from build123d import *

# Parameters (mm, degrees)
BOSS_EXTRUDE1_DEPTH = 4.4
SKETCH2_R           = 3.5
CUT_EXTRUDE1_DEPTH  = 1
SKETCH2_3_R         = 1.7
CUT_EXTRUDE2_DEPTH  = 35.625460286
BOSS_EXTRUDE2_DEPTH = 11.6
FILLET1_R           = 1
CUT_EXTRUDE3_DEPTH  = 5
SKETCH5_R           = 2.5
CUT_EXTRUDE4_DEPTH  = 11


with BuildPart() as part:
    # Sketch1 → Boss-Extrude1 (new body)
    with BuildSketch(Plane(origin=(0, 0, 0), x_dir=(1, 0, 0), z_dir=(0, 1, 0))):
        with BuildLine():
            Line((-11.25, 18), (11.25, 18))
            ThreePointArc((11.25, 18), (29.25, 0), (11.25, -18))
            Line((11.25, -18), (-11.25, -18))
            ThreePointArc((-11.25, -18), (-29.25, 0), (-11.25, 18))
        make_face()
    extrude(amount=BOSS_EXTRUDE1_DEPTH)

    # Sketch2 → Cut-Extrude1 (cut)
    with BuildSketch(Plane(origin=(0, 4.4, 0), x_dir=(1, 0, 0), z_dir=(0, 1, 0))):
        with Locations(Location((-24.25, 0, 0), (0, 0, 270))):
            Circle(SKETCH2_R)
        with Locations(Location((-11.25, 13, 0), (0, 0, 270))):
            Circle(SKETCH2_R)
        with Locations(Location((11.25, 13, 0), (0, 0, 270))):
            Circle(SKETCH2_R)
        with Locations(Location((24.25, 0, 0), (0, 0, 270))):
            Circle(SKETCH2_R)
        with Locations(Location((11.25, -13, 0), (0, 0, 270))):
            Circle(SKETCH2_R)
        with Locations(Location((-11.25, -13, 0), (0, 0, 270))):
            Circle(SKETCH2_R)
    extrude(amount=-CUT_EXTRUDE1_DEPTH, mode=Mode.SUBTRACT)

    # Sketch2<3> → Cut-Extrude2 (cut, through all)
    with BuildSketch(Plane(origin=(0, 4.4, 0), x_dir=(1, 0, 0), z_dir=(0, 1, 0))):
        with Locations(Location((-11.25, 13, 0), (0, 0, 270))):
            Circle(SKETCH2_3_R)
        with Locations(Location((-24.25, 0, 0), (0, 0, 270))):
            Circle(SKETCH2_3_R)
        with Locations(Location((-11.25, -13, 0), (0, 0, 270))):
            Circle(SKETCH2_3_R)
        with Locations(Location((11.25, -13, 0), (0, 0, 270))):
            Circle(SKETCH2_3_R)
        with Locations(Location((24.25, 0, 0), (0, 0, 270))):
            Circle(SKETCH2_3_R)
        with Locations(Location((11.25, 13, 0), (0, 0, 270))):
            Circle(SKETCH2_3_R)
    extrude(amount=-CUT_EXTRUDE2_DEPTH, mode=Mode.SUBTRACT)

    # Sketch3 → Boss-Extrude2 (add)
    with BuildSketch(Plane(origin=(0, 4.4, 0), x_dir=(1, 0, 0), z_dir=(0, 1, 0))):
        with BuildLine():
            Line((-11.25, 7.6), (11.25, 7.6))
            ThreePointArc((11.25, 7.6), (18.85, 0), (11.25, -7.6))
            Line((11.25, -7.6), (-11.25, -7.6))
            ThreePointArc((-11.25, -7.6), (-18.85, 0), (-11.25, 7.6))
        make_face()
    extrude(amount=BOSS_EXTRUDE2_DEPTH)

    # Fillet1
    fillet1_edges = [part.edges().sort_by_distance(p)[0] for p in [
        (29.25, 4.4, 0),
        (0, 4.4, -18),
        (-29.25, 4.4, 0),
        (-18.85, 4.4, 0),
        (0, 4.4, 7.6),
        (18.85, 4.4, 0),
        (0, 4.4, -7.6),
        (0, 4.4, 18),
    ]]
    fillet(fillet1_edges, radius=FILLET1_R)

    # Sketch4 → Cut-Extrude3 (cut)
    with BuildSketch(Plane(origin=(0, 16, 0), x_dir=(1, 0, 0), z_dir=(0, 1, 0))):
        with BuildLine():
            Line((-11.25, 5), (11.25, 5))
            ThreePointArc((11.25, 5), (16.25, 0), (11.25, -5))
            Line((11.25, -5), (-11.25, -5))
            ThreePointArc((-11.25, -5), (-16.25, 0), (-11.25, 5))
        make_face()
    extrude(amount=-CUT_EXTRUDE3_DEPTH, mode=Mode.SUBTRACT)

    # Sketch5 → Cut-Extrude4 (cut)
    with BuildSketch(Plane(origin=(0, 11, 0), x_dir=(1, 0, 0), z_dir=(0, 1, 0))):
        with Locations(Location((-11.25, 0, 0), (0, 0, 270))):
            Circle(SKETCH5_R)
        with Locations(Location((11.25, 0, 0), (0, 0, 270))):
            Circle(SKETCH5_R)
    extrude(amount=-CUT_EXTRUDE4_DEPTH, mode=Mode.SUBTRACT)


solid = part.part
Input: part model. Units: mm. Frame: model coordinates. A direction names the side the tool comes from. Round coordinates to 2 decimals unless told otherwise and drop trailing zeros. Loops run counter-clockwise (first coordinate to the right, second up) from the corner with the lowest first, then second, coordinate; pieces in that order, holes last. Notation, with made-up numbers: (58.5, 59) -> (85.5, 59) arc R16 cw to (85.5, 72) -> close; hole circle Ø11 at (34.5, -16). An arc over 180 degrees is marked (long way). Answer as a JSON object with one key per item and string values. Group by question number.
1) Section query B-B on y = 9.25. Output: boundary loops of the cut face in (x, z), plus the area to 3 significant figures.
2) Draft query along Z for faces 1 (the cylindrical face through (18.85, 10.63, -0.17)), 2 (the cylindrical face through (-14.667, 3.907, -13.759)), 3 (the flat face through (0, 2, 18)). Return one class per face: +Z half, -Z half, draft (parallel to the pull), parting line (faces both ways), or undercut.
3) Ray query, L1, parallel to X at y = 4.15, z = -13; L2, parallel to X at y = 1.5, z = 13; L3, parallel to Z at x = -18, y = 6.75. Return the intervals inside material, ascending.
4) Reachability of faces 4 (the flat face through (0, 11, -7.6)), 5 (the cylindrical face through (25.936, 1.724, -0.221)), 6 (the cylindrical face through (-18.85, 10.63, 0.17)), 7 (the cylindrical face through (-20.78, 3.91, -0.46)) from +Z, -Z, +X, -X, +Y, -Y: full face, straight path, thin tool, end or side. Return the list, or none.
5) Section query C-C on z = 0. State how many separate pieces and enclosed holes the cut face has, plus the area to 3 significant figures.
6) Section query A-A on x = -7. Output: boundary loops of the cut face in (y, z), plus the area to 3 significant figures.
7) Pin query (flat end, axial travel): pin 1 (4 mm diameter, centred on x = -4, y = 13, fed in from +Z); pin 2 (8 mm diameter, centred on y = 8, z = -12.5, fed in from -X); pin 3 (9 mm diameter, centred on x = -24.25, z = 0, fed in from +Y) (3 decimals). Return the tip coordinate at first contact, or that it passes through.
Reply:
{
 "1": {"outline": "(-11.25, -7.6) -> (11.25, -7.6) arc R7.6 ccw to (11.25, 7.6) -> (-11.25, 7.6) arc R7.6 ccw to start; hole circle Ø5 at (-11.25, 0); hole circle Ø5 at (11.25, 0)", "area": "484 mm2"},
 "2": {"face 1": "parting line", "face 2": "undercut", "face 3": "+Z half"},
 "3": {"L1": "x = -23.21 to -14.75, -7.75 to 7.75, 14.75 to 23.21", "L2": "x = -23.7 to -12.95, -9.55 to 9.55, 12.95 to 23.7", "L3": "z = -3.49 to 3.49"},
 "4": {"face 4": "-Z, +X, -X, +Y", "face 5": "+Y, -Y", "face 6": "-X, +Y", "face 7": "+Y"},
 "5": {"separate pieces": "5", "enclosed holes": "0", "area": "385 mm2"},
 "6": {"outline": "(0, -18) -> (3.4, -18) arc R1 ccw to (4.4, -17) -> (4.4, -8.6) arc R1 cw to (5.4, -7.6) -> (16, -7.6) -> (16, -5) -> (11, -5) -> (11, 5) -> (16, 5) -> (16, 7.6) -> (5.4, 7.6) arc R1 cw to (4.4, 8.6) -> (4.4, 17) arc R1 ccw to (3.4, 18) -> (0, 18) -> close", "area": "285 mm2"},
 "7": {"pin 1": "stops at z = 7.6", "pin 2": "stops at x = -24.81", "pin 3": "stops at y = 4.405"}
}
